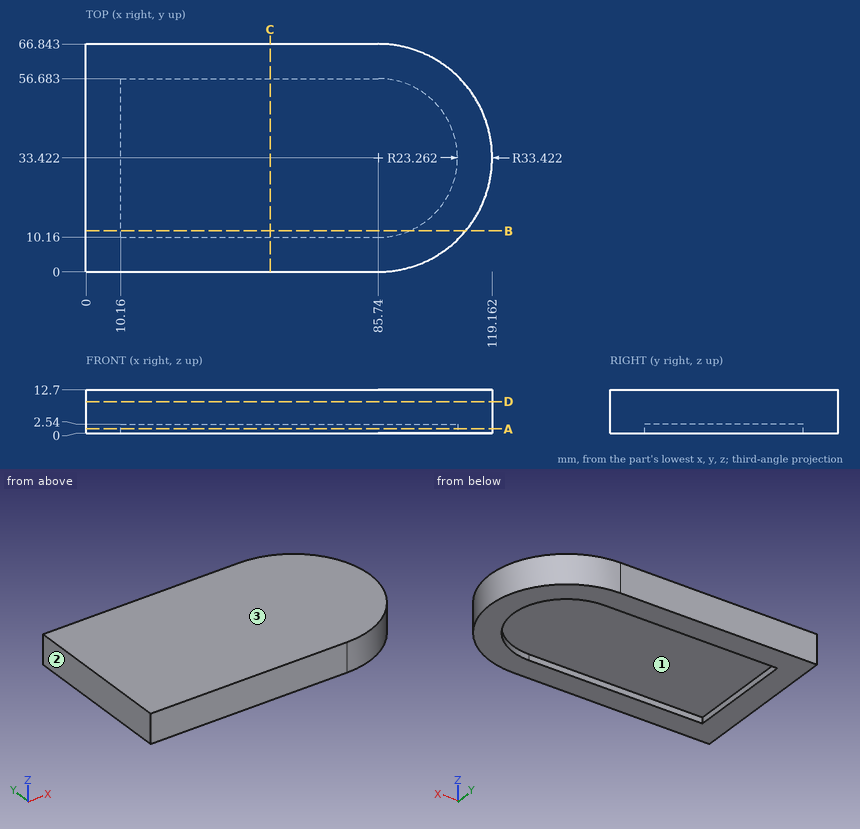
Print and shaded views of the part. All mm, measured from the part's lowest x, y and z. Give positions to 0.01 mm unless a question says otherwise; leave off trailing zeros. Write each loop counter-clockwise with the first axis right and the second up, starting at its lowest first coordinate (ties: lowest second). Pieces come first, ordered by that corner, then holes. Notation, with made-up numbers: (22, 81.5) - (65, 81.5) arc R19 ccw to (65, 93.5) - close; hole circle Ø3 at (-19.5, -33). An arc over 180 degrees is marked (long way). One line per question, with ' | ' between items. Start each with the question number.
(1) Slice it at C-C on x = 54. Write the cut outline in (y, z), plus the area to 3 significant figures.
(2) Wall check: line 1 along Y through (x, z) = (69, 2.5); line 2 along Z through (x, y) = (50, 55); line 3 along X through (y, z) = (61.5, 11.5) (1 decimal). Give the ranges that are in metal, low to high. Write a range as from..to.
(3) Slice it at B-B on y = 12. Write the cut outline in (x, z) (1 decimal).
(4) Slice it at A-A on z = 1.25. Write the cut outline in (x, y), plus the area to 3 significant figures.
(5) Pin check, flat tips, straight feed: P1, Ø1.5, axis at x = 60, z = 7, coming from the -Y side; P2, Ø3, axis at y = 11.5, z = 10, coming from the +X side; P3, Ø1, axis at x = 41, y = 27, coming from the -Z side; P4, Ø1.3, axis at y = 36.5, z = 1, coming from the +X side. Stop position of each tip, or through.
(6) Two-plate mould, pull along X, no slides. Class the marked faces 1, 2 and 3: +X half, -X half, draft (parallel to the pull), parting line (faces both ways), or undercut.
(7) Slice it at D-D on z = 9.25. Write the cut outline in (x, y).
Results below:
1) outline: (0, 0) - (10.16, 0) - (10.16, 2.54) - (56.68, 2.54) - (56.68, 0) - (66.84, 0) - (66.84, 12.7) - (0, 12.7) - close | area: 731 mm^2
2) line 1: 0..10.16, 56.68..66.84 | line 2: 2.54..12.7 | line 3: 0..103.9
3) outline: (0, 0) - (10.2, 0) - (10.2, 2.5) - (94.8, 2.5) - (94.8, 0) - (111.4, 0) - (111.4, 12.7) - (0, 12.7) - close
4) outline: (0, 0) - (85.74, 0) arc R33.42 ccw to (85.74, 66.84) - (0, 66.84) - close; hole (10.16, 10.16) - (85.74, 10.16) arc R23.26 ccw to (85.74, 56.68) - (10.16, 56.68) - close | area: 3,120 mm^2
5) P1: y = 0 | P2: x = 112.2 | P3: z = 2.54 | P4: x = 119.07
6) face 1: undercut | face 2: -X half | face 3: draft
7) outline: (0, 0) - (85.74, 0) arc R33.42 ccw to (85.74, 66.84) - (0, 66.84) - close
